from build123d import *

# Parameters (mm, degrees)
SKETCH1_W           = 12
SKETCH1_H           = 25.2
BOSS_EXTRUDE1_DEPTH = 3
FILLET1_R           = 6
SKETCH3_W           = 12
SKETCH3_H           = 20
BOSS_EXTRUDE2_DEPTH = 2
FILLET2_R           = 6
CUT_EXTRUDE1_DEPTH  = 3
SKETCH5_R           = 2.8
CUT_EXTRUDE2_DEPTH  = 126.573231257
SKETCH6_R           = 1
CUT_EXTRUDE3_DEPTH  = 126.573231257
SKETCH7_W           = 12.403914783
SKETCH7_H           = 13.383655683
CUT_EXTRUDE4_DEPTH  = 1
FILLET3_R           = 1.5


with BuildPart() as part:
    # Sketch1 → Boss-Extrude1 (new body)
    with BuildSketch(Plane.XY.offset(5)):
        with Locations((-54.027704131, 97.655662644)):
            Rectangle(SKETCH1_W, SKETCH1_H)
    extrude(amount=BOSS_EXTRUDE1_DEPTH)

    # Fillet1
    fillet1_edges = [part.edges().sort_by_distance(p)[0] for p in [
        (-48.027704131, 85.055662644, 6.5),
        (-60.027704131, 85.055662644, 6.5),
    ]]
    fillet(fillet1_edges, radius=FILLET1_R - 0.0001)  # a hair under: the kernel refuses the full size

    # Sketch3 → Boss-Extrude2 (add)
    with BuildSketch(Plane.XY.offset(8)):
        with Locations((-54.027704131, 95.017998247)):
            Rectangle(SKETCH3_W, SKETCH3_H)
    extrude(amount=BOSS_EXTRUDE2_DEPTH)

    # Fillet2
    fillet2_edges = [part.edges().sort_by_distance(p)[0] for p in [
        (-48.027704131, 85.017998247, 9),
        (-60.027704131, 85.017998247, 9),
    ]]
    fillet(fillet2_edges, radius=FILLET2_R - 0.0001)  # a hair under: the kernel refuses the full size

    # Sketch4 → Cut-Extrude1 (cut, symmetric)
    with BuildSketch(Plane.XY.offset(10)):
        with BuildLine():
            Line((-56.13842392, 104.48600769), (-51.86157608, 104.48600769))
            Line((-51.86157608, 104.48600769), (-50.824897766, 90.586959839))
            ThreePointArc((-50.824897766, 90.586959839), (-54.164460237, 87.789583498), (-57.199226379, 90.914993286))
            Line((-57.199226379, 90.914993286), (-56.13842392, 104.48600769))
        make_face()
    extrude(amount=CUT_EXTRUDE1_DEPTH, both=True, mode=Mode.SUBTRACT)

    # Sketch5 → Cut-Extrude2 (cut, through all)
    with BuildSketch(Plane.XY.offset(7)):
        with Locations((-53.997448325, 91.08203191)):
            Circle(SKETCH5_R)
    extrude(amount=-CUT_EXTRUDE2_DEPTH, mode=Mode.SUBTRACT)

    # Sketch6 → Cut-Extrude3 (cut, through all)
    with BuildSketch(Plane.XY.offset(8)):
        with Locations((-57.999885247, 107.886757068)):
            Circle(SKETCH6_R)
        with Locations((-49.934118523, 107.886757068)):
            Circle(SKETCH6_R)
    extrude(amount=-CUT_EXTRUDE3_DEPTH, mode=Mode.SUBTRACT)

    # Sketch7 → Cut-Extrude4 (cut)
    with BuildSketch(Plane.XY.offset(10)):
        with Locations((-53.82574674, 91.326170406)):
            Rectangle(SKETCH7_W, SKETCH7_H)
    extrude(amount=-CUT_EXTRUDE4_DEPTH, mode=Mode.SUBTRACT)

    # Fillet3
    fillet3_edges = [part.edges().sort_by_distance(p)[0] for p in [
        (-60.027704131, 110.255662644, 6.5),
        (-48.027704131, 110.255662644, 6.5),
    ]]
    fillet(fillet3_edges, radius=FILLET3_R)


solid = part.part
Model file for the job. Use its own axes, mm. A direction names the side the tool comes from. Coordinates: 2 decimals unless noted, no trailing zeros. Order: outer loops, then holes, each group sorted by start corner. A loop starts at its lowest first (then second) coordinate and runs counter-clockwise, first axis right, second up. Notation, with made-up numbers: M 1.25,-18 L 35.25,-18 A9 ccw 35.25,-11 Z; hole C -31.75,89 d1. An arc over 180 degrees is marked long. Return JSON: item names as keys, results as strings.
1. Tool access for faces 1 (the face through (-58.317, 86.86, 6.521)), 2 (the face through (-49.8, 86.8, 6.5)), 3 (the face through (-54, 98, 5)), 4 (the face through (-54, 108, 8)), 5 (the face through (-51.35, 97.63, 8.19)): list every direction of +Z, -Z, +X, -X, +Y, -Y with a clear straight run to the whole face (end or side of a thin tool).
Ans:
{"face 1": "-Z, -X, -Y", "face 2": "-Z, +X, -Y", "face 3": "-Z, +X, -X, +Y, -Y", "face 4": "+Z, +X, -X, +Y", "face 5": "+Z"}
2. Saw through at C-C (y = 92.5). Give the cut face in (x, z), and give its area (3 significant figures).
Ans:
{"outline": "M -60.03,5 L -56.41,5 L -56.41,7 L -57.08,7 L -57.08,9 L -60.03,9 Z; M -51.58,5 L -48.03,5 L -48.03,9 L -50.97,9 L -50.97,7 L -51.58,7 Z", "area": "26.1 mm^2"}
3. Saw through at D-D (z = 6.3). Give the number of separate pieces and of enclosed holes in the cut face, and give its area (3 significant figures).
Ans:
{"separate pieces": "1", "enclosed holes": "3", "area": "255 mm^2"}
4. Flat gauge pins, fed straight in: pin 1 (1.8 mm diameter, centred on x = -58, y = 107.89, fed in from -Z); pin 2 (0.8 mm diameter, centred on x = -50, z = 9.5, fed in from -Y); pin 3 (2 mm diameter, centred on y = 89, z = 6, fed in from +X); pin 4 (6 mm diameter, centred on x = -54, y = 89, fed in from +Z). Where does each tip first touch, or does it go through?
Ans:
{"pin 1": "through", "pin 2": "y = 98.02", "pin 3": "x = -48.12", "pin 4": "z = 9"}
5. Drill centre lines: probe 1 along Z at (x, y) = (-49.75, 88); probe 2 along X at (y, z) = (90.25, 7.4); probe 3 along Y at (x, z) = (-53.5, 5.9). Where is each one in solid material? Low to high.
Ans:
{"probe 1": "5 to 9", "probe 2": "-59.97 to -57.11, -50.89 to -48.08", "probe 3": "85.08 to 88.33, 93.84 to 110.26"}
6. Pull direction X, two halves, no side cores. Call faces 6 (the face through (-49.7, 98.018, 9.5)), 7 (the face through (-48.48, 109.83, 6.52)), 8 (the face through (-56.676, 97.606, 8.188)): +X half, -X half, draft (parallel to the pull), parting line (faces both ways), or undercut.
Ans:
{"face 6": "draft", "face 7": "+X half", "face 8": "undercut"}
